The listing builds one solid part. Answer for the finished solid, in the listing's coordinates (mm). Give positions to 0.01 mm unless a question says otherwise; leave off trailing zeros. Write each loop counter-clockwise with the first axis right and the second up, starting at its lowest first coordinate (ties: lowest second). Pieces come first, ordered by that corner, then holes. Notation, with made-up numbers: M -29.5,85.25 L 2.5,85.25 A31 ccw 2.5,111.25 Z; hole C 0,-20 d1. An arc over 180 degrees is marked long. Return JSON: item names as keys, results as strings.
Autodesk Inventor part; units mm, degrees
ref_plane "YZ Plane" through (0, 0, 0) normal (1, 0, 0) x (0, 1, 0)
ref_plane "XZ Plane" through (0, 0, 0) normal (0, 1, 0) x (-1, 0, 0)
ref_plane "XY Plane" through (0, 0, 0) normal (0, 0, 1) x (1, 0, 0)
sketch "スケッチ1" plane through (0, 0, 0) normal (0, 0, 1) x (1, 0, 0)
  circle A0 centre (-149.101, -13.3308) radius 1.5 construction
  circle A1 centre (-160.5892, -1.6149) radius 1.5 construction
  circle A2 centre (-44.4492, 64.0137) radius 1.5 construction
  circle A3 centre (-64.4423, 49.0046) radius 1.5 construction
  circle A4 centre (-60.4494, 64.5064) radius 1.5 construction
  arc A5 (-40.2316, 58.3956) -> (-44.233, 71.0354) centre (-44.4492, 64.0137) ccw construction
  line L0 (-44.233, 71.0354) -> (-60.2332, 71.5281) construction
  arc A6 (-60.2332, 71.5281) -> (-64.1725, 70.4637) centre (-60.4494, 64.5064) ccw construction
  line L1 (-64.1725, 70.4637) -> (-165.9022, 6.8864) construction
  arc A7 (-165.9022, 6.8864) -> (-166.8262, -9.4635) centre (-160.5892, -1.6149) ccw construction
  line L2 (-166.8262, -9.4635) -> (-154.0782, -19.594) construction
  arc A8 (-154.0782, -19.594) -> (-144.2981, -19.7286) centre (-149.101, -13.3308) ccw construction
  line L3 (-144.2981, -19.7286) -> (-40.2316, 58.3956) construction
  circle A9 centre (-82.1645, 51.5544) radius 1.5 construction
  circle A10 centre (-141.748, 14.817) radius 1.5 construction
  circle A11 centre (-89.4637, 29.5642) radius 1.5 construction
  circle A12 centre (-117.4541, 8.5514) radius 1.5 construction
  circle A13 centre (-111.8449, 33.0052) radius 1.5 construction
  line L4 (-152.7009, -26.0367) -> (-305.9655, -141.0946)
  circle A14 centre (-149.101, -13.3308) radius 1.5 construction
  circle A15 centre (-149.101, -13.3308) radius 3 construction
  circle A16 centre (-149.101, -13.3308) radius 3 construction
  circle A17 centre (-160.5892, -1.6149) radius 9.025 construction
  circle A18 centre (-160.5892, -1.6149) radius 4.025
  line L5 (-152.7009, -26.0367) -> (-151.5741, -2.0382)
  line L6 (-64.1725, 70.4637) -> (-165.9022, 6.8864) construction
  line L7 (-144.2981, -19.7286) -> (-40.2316, 58.3956) construction
  line L8 (-305.9655, -141.0946) -> (-171.4423, -28.6314)
  line L9 (-160.5892, -1.6149) -> (-146.0204, -21.0215) construction
  line L10 (-146.0204, -21.0215) -> (-305.9655, -141.0946) construction
  circle A19 centre (-276.0256, -117.3678) radius 1
  circle A20 centre (-160.5892, -1.6149) radius 11
  line L11 (-171.4423, -28.6314) -> (-171.589, -1.6748)
  point P0 (0, 0)
  point P1 (0, 0)
  point P2 (0, 0)
  point P3 (-276.667, -116.6006)
  point P4 (-275.4252, -118.1676)
  point P5 (-151.8691, -8.3201)
  dimension "d6" = 22
  dimension "d0" = 6
  dimension "d1" = 8.05
  dimension "d2" = 5
  dimension "d3" = 3
  dimension "d4" = 200
  dimension "d5" = 2
  dimension "d7" = 3
  dimension "d8" = 6
sketch "スケッチ2" plane through (0, 0, 0) normal (0, 0, 1) x (1, 0, 0)
  line L0 (-305.9655, -141.0946) -> (-171.4423, -28.6314)
  line L1 (-171.4423, -28.6314) -> (-171.589, -1.6748)
  line L2 (-302.5902, -138.2728) -> (-303.873, -136.7384)
  line L3 (-303.873, -136.7384) -> (-173.4475, -27.7009)
  line L4 (-173.4475, -27.7009) -> (-173.9864, 71.3562)
  line L5 (-173.9864, 71.3562) -> (-171.9864, 71.3671)
  line L6 (-171.9864, 71.3671) -> (-171.589, -1.6748)
  point P0 (0, 0)
  dimension "d9" = 2
  dimension "d10" = 2
  dimension "d11" = 100
  dimension "d14" = 170
extrude "押し出し1" add sketch "スケッチ2" along normal blind 270
sketch "スケッチ3" plane through (0, 0, 270) normal (0, 0, 1) x (1, 0, 0)
  arc A0 (-225.7, -73.9915) -> (-224.5724, -73.0489) centre (-225.6172, -72.9448) ccw
  line L0 (-225.7, -73.9915) -> (-243.7526, -89.0838)
  arc A1 (-244.8802, -90.0264) -> (-243.7526, -89.0838) centre (-244.7975, -88.9797) ccw
  line L1 (-244.8802, -90.0264) -> (-276.667, -116.6006)
  arc A2 (-276.667, -116.6006) -> (-275.4252, -118.1676) centre (-276.0256, -117.3678) ccw
  line L2 (-275.4252, -118.1676) -> (-152.7009, -26.0367)
  line L3 (-152.7009, -26.0367) -> (-151.8691, -8.3201)
  arc A3 (-151.8691, -8.3201) -> (-171.589, -1.6748) centre (-160.5892, -1.6149) ccw
  line L4 (-171.589, -1.6748) -> (-171.4423, -28.6314)
  line L5 (-171.4423, -28.6314) -> (-186.2119, -40.979)
  arc A4 (-187.3395, -41.9217) -> (-186.2119, -40.979) centre (-187.2568, -40.8749) ccw
  line L6 (-187.3395, -41.9217) -> (-205.3922, -57.0139)
  arc A5 (-206.5197, -57.9566) -> (-205.3922, -57.0139) centre (-206.437, -56.9099) ccw
  line L7 (-206.5197, -57.9566) -> (-224.5724, -73.0489)
  circle A6 centre (-171.2358, -34.3242) radius 1.5
  circle A7 centre (-160.5892, -1.6149) radius 4.025
  point P0 (0, 0)
  point P1 (0, 0)
sketch "スケッチ4" plane through (-303.873, -136.7384, 270) normal (-0.6413971, 0.7672091, 0) x (0.7672091, 0.6413971, 0)
  line L0 (234.6628, 270) -> (234.6628, 0)
  circle A0 centre (150.9556, 102) radius 1.5
  circle A1 centre (125.9556, 102) radius 1.5
  circle A2 centre (100.9556, 102) radius 1.5
  circle A3 centre (75.9556, 102) radius 1.5
  line L1 (234.6628, 135) -> (-10.981, 135)
  circle A4 centre (150.9556, 168) radius 1.5
  circle A5 centre (125.9556, 168) radius 1.5
  circle A6 centre (100.9556, 168) radius 1.5
  circle A7 centre (75.9556, 168) radius 1.5
  line L2 (154.7693, 165) -> (132.5454, 165)
  line L3 (157.7493, 105) -> (143.6573, 105)
  point P0 (320.8377, 270)
  point P1 (150.9556, 0)
  point P2 (125.9556, 0)
  point P3 (100.9556, 0)
  point P4 (75.9556, 0)
  dimension "d15" = 3
  dimension "d16" = 3
  dimension "d17" = 3
  dimension "d18" = 3
  dimension "d20" = 33
  dimension "d27" = 3
  dimension "d28" = 3
  dimension "d29" = 60
extrude "押し出し2" cut sketch "スケッチ4" against normal through all
chamfer "面取り1" distance 100 angle 45 2 edges at (-303.2316, -137.5056, 0) (-303.2316, -137.5056, 270)
sketch "スケッチ5" plane through (-171.9864, 71.3671, 270) normal (0.9999852, 0.0054408, 0) x (0, 0, -1)
  line L0 (270, 0) -> (0, 0)
  line L1 (0, 0) -> (0, -99.0586)
  line L2 (0, 0) -> (25, 0)
  line L3 (270, 0) -> (245, 0)
  line L4 (245, 0) -> (245, -20)
  line L5 (245, -20) -> (25, -20)
  line L6 (25, -20) -> (25, 0)
  point P0 (270, -72.3018)
  dimension "d30" = 25
  dimension "d31" = 25
  dimension "d32" = 20
extrude "押し出し3" cut sketch "スケッチ5" against normal through all
equation "\"d8\" = d0"
properties part number "アームシールド1" material "ポリカーボネート、クリア"
Item 1: A cutting plane is placed at D-D, the plane z = 39. Write down the section's boundary in (x, y), plus the area to 3 significant figures.
Geometry results:
{"outline": "M -257.07,-97.61 L -255.79,-99.15 L -171.44,-28.63 L -171.59,-1.67 L -171.88,51.37 L -173.88,51.36 L -173.45,-27.7 Z", "area": "378 mm2"}
Item 2: Given pin 1 Ø12 at (y, z) = (-83, 158) entering from +X; pin 2 Ø8 at (x, z) = (-198, 76.5) entering from -Y; pin 3 Ø2 at (x, z) = (-252, 242) entering from +Y; pin 4 Ø2 at (y, z) = (-54, 234) entering from -X, each flat-ended and moving along its own axis, determine where each tip first touches the part or whether it passes through.
Geometry results:
{"pin 1": "stops at x = -229.3", "pin 2": "stops at y = -54.18", "pin 3": "passes through", "pin 4": "stops at x = -206.1"}
Item 3: Find the intervals of material crossed by line 1 (Z direction, x = -245.5, y = -90); line 2 (X direction, y = 26.5, z = 167); line 3 (X direction, y = -14.5, z = 117.5), in increasing order.
Geometry results:
{"line 1": "z = 25.24 to 101.09, 102.91 to 167.09, 168.91 to 244.76", "line 2": "x = -173.74 to -171.74", "line 3": "x = -173.52 to -171.52"}
Item 4: A cutting plane is placed at C-C, the plane y = -10.5. Write down the section's boundary in (x, z), plus the area to 3 significant figures.
Geometry results:
{"outline": "M -173.54,0 L -171.54,0 L -171.54,270 L -173.54,270 Z", "area": "540 mm2"}
Item 5: A cutting plane is placed at B-B, the plane x = -276.5. Write down the section's boundary in (y, z), plus the area to 3 significant figures.
Geometry results:
{"outline": "M -116.46,65.99 L -113.85,64.32 L -113.85,205.68 L -116.46,204.01 Z", "area": "364 mm2"}
Item 6: A cutting plane is placed at A-A, the plane z = 157.5. Write down the section's boundary in (x, y).
Geometry results:
{"outline": "M -303.87,-136.74 L -302.59,-138.27 L -171.44,-28.63 L -171.59,-1.67 L -171.88,51.37 L -173.88,51.36 L -173.45,-27.7 Z"}
